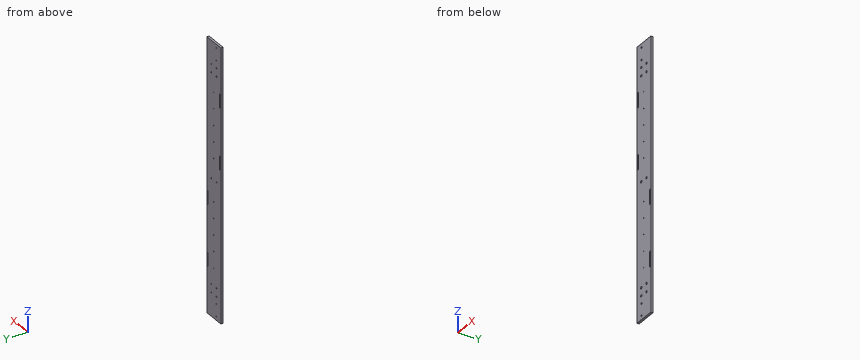
from build123d import *

# Parameters (mm, degrees)
SKETCH_1_W                  = 80
SKETCH_1_H                  = 8
EXTRUDE_1_DEPTH             = 1000
SKETCH_3_R                  = 4
CUT_EXTRUDE_1_DEPTH         = 5
SKETCH_4_R                  = 2.25
CUT_EXTRUDE_2_DEPTH         = 5
SKETCH_5_R                  = 2.25
CUT_EXTRUDE_3_DEPTH         = 8
PATTERN_LINEAR_1_COUNT      = 2
PATTERN_LINEAR_1_PITCH      = 30
PATTERN_LINEAR_1_COUNT_DIR2 = 2
PATTERN_LINEAR_1_PITCH_DIR2 = 30
SKETCH_6_R                  = 4
CUT_EXTRUDE_4_DEPTH         = 5
PATTERN_LINEAR_2_COUNT      = 2
PATTERN_LINEAR_2_PITCH      = 30
PATTERN_LINEAR_2_COUNT_DIR2 = 2
PATTERN_LINEAR_2_PITCH_DIR2 = 30
SKETCH_7_R                  = 2.25
CUT_EXTRUDE_5_DEPTH         = 8
PATTERN_LINEAR_3_COUNT      = 2
PATTERN_LINEAR_3_PITCH      = 30
PATTERN_LINEAR_3_COUNT_DIR2 = 2
PATTERN_LINEAR_3_PITCH_DIR2 = 30
SKETCH_8_R                  = 4
CUT_EXTRUDE_6_DEPTH         = 5
PATTERN_LINEAR_4_COUNT      = 2
PATTERN_LINEAR_4_PITCH      = 30
PATTERN_LINEAR_4_COUNT_DIR2 = 2
PATTERN_LINEAR_4_PITCH_DIR2 = 30
CUT_EXTRUDE_8_DEPTH         = 4
CUT_EXTRUDE_9_DEPTH         = 5
PATTERN_LINEAR_6_COUNT      = 2
PATTERN_LINEAR_6_PITCH      = 225
PATTERN_LINEAR_6_COL_COUNT  = 2
PATTERN_LINEAR_6_COL_PITCH  = 225
SKETCH_13_R                 = 1.5
CUT_EXTRUDE_10_DEPTH        = 8
SKETCH_14_R                 = 3
CUT_EXTRUDE_11_DEPTH        = 4
PATTERN_LINEAR_8_COUNT      = 2
PATTERN_LINEAR_8_PITCH      = 927
SKETCH_15_R                 = 1.65
CUT_EXTRUDE_12_DEPTH        = 10
PATTERN_LINEAR_9_COUNT      = 5
PATTERN_LINEAR_9_PITCH      = 60
SKETCH_16_R                 = 1.65
CUT_EXTRUDE_13_DEPTH        = 10
PATTERN_LINEAR_10_COUNT     = 5
PATTERN_LINEAR_10_PITCH     = 60


with BuildPart() as part:
    # Эскиз1 → Бобышка-Вытянуть1 (new body)
    with BuildSketch(Plane.XY):
        Rectangle(SKETCH_1_W, SKETCH_1_H)
    extrude(amount=EXTRUDE_1_DEPTH)

    # Эскиз3 → Вырез-Вытянуть1 (cut)
    with BuildSketch(Plane.XZ.offset(4)):
        with Locations(Location((15, 500, 0), (0, 0, 270))):
            Circle(SKETCH_3_R)
        with Locations(Location((-15, 500, 0), (0, 0, 270))):
            Circle(SKETCH_3_R)
    extrude(amount=-CUT_EXTRUDE_1_DEPTH, mode=Mode.SUBTRACT)

    # Эскиз4 → Вырез-Вытянуть2 (cut)
    with BuildSketch(Plane.XZ.offset(-1)):
        with Locations(Location((-15, 500, 0), (0, 0, 270))):
            Circle(SKETCH_4_R)
        with Locations(Location((15, 500, 0), (0, 0, 270))):
            Circle(SKETCH_4_R)
    extrude(amount=-CUT_EXTRUDE_2_DEPTH, mode=Mode.SUBTRACT)

    # Эскиз5 → Вырез-Вытянуть3 (cut)
    with BuildSketch(Plane.XZ.offset(4)):
        with Locations(Location((-15, 913.6, 0), (0, 0, 270))):
            Circle(SKETCH_5_R)
    cut_extrude_3 = extrude(amount=-CUT_EXTRUDE_3_DEPTH, mode=Mode.SUBTRACT)

    # Линейный массив1: Cut-Extrude 3 2 × 2
    with Locations(*[(i * PATTERN_LINEAR_1_PITCH, 0, -j * PATTERN_LINEAR_1_PITCH_DIR2) for i in range(PATTERN_LINEAR_1_COUNT) for j in range(PATTERN_LINEAR_1_COUNT_DIR2) if (i, j) != (0, 0)]):
        add(cut_extrude_3, mode=Mode.SUBTRACT)

    # Эскиз6 → Вырез-Вытянуть4 (cut)
    with BuildSketch(Plane.XZ.offset(4)):
        with Locations(Location((-15, 913.6, 0), (0, 0, 270))):
            Circle(SKETCH_6_R)
    cut_extrude_4 = extrude(amount=-CUT_EXTRUDE_4_DEPTH, mode=Mode.SUBTRACT)

    # Линейный массив2: Cut-Extrude 4 2 × 2
    with Locations(*[(i * PATTERN_LINEAR_2_PITCH, 0, -j * PATTERN_LINEAR_2_PITCH_DIR2) for i in range(PATTERN_LINEAR_2_COUNT) for j in range(PATTERN_LINEAR_2_COUNT_DIR2) if (i, j) != (0, 0)]):
        add(cut_extrude_4, mode=Mode.SUBTRACT)

    # Эскиз7 → Вырез-Вытянуть5 (cut)
    with BuildSketch(Plane.XZ.offset(4)):
        with Locations(Location((-15, 86.4, 0), (0, 0, 270))):
            Circle(SKETCH_7_R)
    cut_extrude_5 = extrude(amount=-CUT_EXTRUDE_5_DEPTH, mode=Mode.SUBTRACT)

    # Линейный массив3: Cut-Extrude 5 2 × 2
    with Locations(*[(i * PATTERN_LINEAR_3_PITCH, 0, j * PATTERN_LINEAR_3_PITCH_DIR2) for i in range(PATTERN_LINEAR_3_COUNT) for j in range(PATTERN_LINEAR_3_COUNT_DIR2) if (i, j) != (0, 0)]):
        add(cut_extrude_5, mode=Mode.SUBTRACT)

    # Эскиз8 → Вырез-Вытянуть6 (cut)
    with BuildSketch(Plane.XZ.offset(4)):
        with Locations(Location((-15, 86.4, 0), (0, 0, 270))):
            Circle(SKETCH_8_R)
    cut_extrude_6 = extrude(amount=-CUT_EXTRUDE_6_DEPTH, mode=Mode.SUBTRACT)

    # Линейный массив4: Cut-Extrude 6 2 × 2
    with Locations(*[(i * PATTERN_LINEAR_4_PITCH, 0, j * PATTERN_LINEAR_4_PITCH_DIR2) for i in range(PATTERN_LINEAR_4_COUNT) for j in range(PATTERN_LINEAR_4_COUNT_DIR2) if (i, j) != (0, 0)]):
        add(cut_extrude_6, mode=Mode.SUBTRACT)

    # Эскиз11 → Вырез-Вытянуть8 (cut)
    with BuildSketch(Plane.XZ.offset(4)):
        with BuildLine():
            Line((37.5, 220), (37.5, 170))
            ThreePointArc((37.5, 170), (34.5, 167), (31.5, 170))
            Line((31.5, 170), (31.5, 220))
            ThreePointArc((31.5, 220), (34.5, 223), (37.5, 220))
        make_face()
        with BuildLine():
            Line((-31.5, 830), (-31.5, 780))
            ThreePointArc((-31.5, 780), (-34.5, 777), (-37.5, 780))
            Line((-37.5, 780), (-37.5, 830))
            ThreePointArc((-37.5, 830), (-34.5, 833), (-31.5, 830))
        make_face()
    cut_extrude_8 = extrude(amount=-CUT_EXTRUDE_8_DEPTH, mode=Mode.SUBTRACT)

    # Эскиз12 → Вырез-Вытянуть9 (cut)
    with BuildSketch(Plane(origin=(0, 0, 0), x_dir=(-1, 0, 0), z_dir=(0, -1, 0))):
        with BuildLine():
            Line((-36.25, -218.75), (-36.25, -171.25))
            ThreePointArc((-36.25, -171.25), (-34.5, -169.5), (-32.75, -171.25))
            Line((-32.75, -171.25), (-32.75, -218.75))
            ThreePointArc((-32.75, -218.75), (-34.5, -220.5), (-36.25, -218.75))
        make_face()
        with BuildLine():
            Line((32.75, -828.75), (32.75, -781.25))
            ThreePointArc((32.75, -781.25), (34.5, -779.5), (36.25, -781.25))
            Line((36.25, -781.25), (36.25, -828.75))
            ThreePointArc((36.25, -828.75), (34.5, -830.5), (32.75, -828.75))
        make_face()
    cut_extrude_9 = extrude(amount=-CUT_EXTRUDE_9_DEPTH, mode=Mode.SUBTRACT)

    # Линейный массив6: Вырез-Вытянуть8, Вырез-Вытянуть9 ×2
    with Locations(*[(0, 0, i * PATTERN_LINEAR_6_PITCH) for i in range(1, PATTERN_LINEAR_6_COUNT)]):
        add(cut_extrude_8, mode=Mode.SUBTRACT)
        add(cut_extrude_9, mode=Mode.SUBTRACT)

    # Линейный массив6 col: Вырез-Вытянуть8, Вырез-Вытянуть9 ×2
    with Locations(*[(0, 0, -i * PATTERN_LINEAR_6_COL_PITCH) for i in range(1, PATTERN_LINEAR_6_COL_COUNT)]):
        add(cut_extrude_8, mode=Mode.SUBTRACT)
        add(cut_extrude_9, mode=Mode.SUBTRACT)

    # Эскиз13 → Вырез-Вытянуть10 (cut)
    with BuildSketch(Plane.XZ.offset(4)):
        with Locations(Location((-14, 59, 0), (0, 0, 270))):
            Circle(SKETCH_13_R)
        with Locations(Location((-14, 14, 0), (0, 0, 270))):
            Circle(SKETCH_13_R)
    cut_extrude_10 = extrude(amount=-CUT_EXTRUDE_10_DEPTH, mode=Mode.SUBTRACT)

    # Эскиз14 → Вырез-Вытянуть11 (cut)
    with BuildSketch(Plane.XZ.offset(4)):
        with Locations(Location((-14, 59, 0), (0, 0, 270))):
            Circle(SKETCH_14_R)
        with Locations(Location((-14, 14, 0), (0, 0, 270))):
            Circle(SKETCH_14_R)
    cut_extrude_11 = extrude(amount=-CUT_EXTRUDE_11_DEPTH, mode=Mode.SUBTRACT)

    # Линейный массив8: Вырез-Вытянуть10, Вырез-Вытянуть11 ×2
    with Locations(*[(0, 0, i * PATTERN_LINEAR_8_PITCH) for i in range(1, PATTERN_LINEAR_8_COUNT)]):
        add(cut_extrude_10, mode=Mode.SUBTRACT)
        add(cut_extrude_11, mode=Mode.SUBTRACT)

    # Эскиз15 → Вырез-Вытянуть12 (cut)
    with BuildSketch(Plane.XZ.offset(4)):
        with Locations(Location((0, 421.45, 0), (0, 0, 270))):
            Circle(SKETCH_15_R)
    cut_extrude_12 = extrude(amount=-CUT_EXTRUDE_12_DEPTH, mode=Mode.SUBTRACT)

    # Линейный массив9: Вырез-Вытянуть12 ×5
    with Locations(*[(0, 0, -i * PATTERN_LINEAR_9_PITCH) for i in range(1, PATTERN_LINEAR_9_COUNT)]):
        add(cut_extrude_12, mode=Mode.SUBTRACT)

    # Эскиз16 → Вырез-Вытянуть13 (cut)
    with BuildSketch(Plane.XZ.offset(4)):
        with Locations(Location((0, 578.55, 0), (0, 0, 270))):
            Circle(SKETCH_16_R)
    cut_extrude_13 = extrude(amount=-CUT_EXTRUDE_13_DEPTH, mode=Mode.SUBTRACT)

    # Линейный массив10: Вырез-Вытянуть13 ×5
    with Locations(*[(0, 0, i * PATTERN_LINEAR_10_PITCH) for i in range(1, PATTERN_LINEAR_10_COUNT)]):
        add(cut_extrude_13, mode=Mode.SUBTRACT)


solid = part.part
CAD build for the part. Positions are in the model's coordinates, mm. Coordinates: 2 decimals unless noted, no trailing zeros. One line per item, written item: value.
1. Drill centre lines: line 1 (X direction, y = 0.5, z = 181.45); line 2 (X direction, y = 1.4, z = 59); line 3 (X direction, y = -1.75, z = 86.4). Where is each one in solid material? Low to high. Write a range as [from, to].
Answers:
line 1: x = [-40, -1.65], [1.65, 32.75], [36.25, 40]
line 2: x = [-40, -15.5], [-12.5, 40]
line 3: x = [-40, -19], [-11, 11], [19, 40]
2. Slice it at A-A on y = -2.5. Give the number of separate pieces and of enclosed holes in the cut face, and give its area (3 significant figures).
Answers:
separate pieces: 1
enclosed holes: 28
area: 78,000 mm^2
3. Flat gauge pins, fed straight in: P1, Ø7, axis at x = 15, z = 86.4, coming from the -Y side; P2, Ø1.8, axis at x = -13.5, z = 987, coming from the -Y side. Where does each tip first touch, or does it go through?
Answers:
P1: stops at y = 1
P2: stops at y = 0
